from build123d import *

# Parameters (mm, degrees)
SKETCH6_R          = 4.25
CUT_EXTRUDE3_DEPTH = 20.176579466
CUT_EXTRUDE4_DEPTH = 6.35


with BuildPart() as part:
    # Sketch2 → Revolve1 (revolve)
    with BuildSketch(Plane(origin=(0, 0, 0), x_dir=(0, 0, -1), z_dir=(1, 0, 0)), mode=Mode.PRIVATE) as revolve1_sk:
        Polygon((0, 0), (-6.35, 0), (-10.16, -9.525), (-10.16, -12.7), (0, -12.7), align=None)
    revolve(revolve1_sk.sketch.rotate(Axis((0, -12.7, 0), (0, 1, 0)), 180), axis=Axis((0, -12.7, 0), (0, 1, 0)))

    # Sketch6 → Cut-Extrude3 (cut, through all)
    with BuildSketch(Plane(origin=(0, 0, 0), x_dir=(1, 0, 0), z_dir=(0, 1, 0))):
        with Locations(Location((0, 0, 0), (0, 0, 270))):
            Circle(SKETCH6_R)
    extrude(amount=-CUT_EXTRUDE3_DEPTH, mode=Mode.SUBTRACT)

    # Sketch7 → Cut-Extrude4 (cut)
    with BuildSketch(Plane.XZ.offset(12.7)):
        Polygon((0, 7.274613392), (-6.3, 3.637306696), (-6.3, -3.637306696), (0, -7.274613392), (6.3, -3.637306696), (6.3, 3.637306696), align=None)
    extrude(amount=-CUT_EXTRUDE4_DEPTH, mode=Mode.SUBTRACT)


solid = part.part
Verification items for the finished model (mm, model axes). A direction names the side the tool comes from. Give positions to 0.01 mm unless a question says otherwise; leave off trailing zeros. Loops run counter-clockwise (first coordinate to the right, second up) from the corner with the lowest first, then second, coordinate; pieces in that order, holes last.
1) Depth check by flat-ended pin: pin 1 Ø2 at (x, y) = (3, -3) entering from +Z; pin 2 Ø2 at (x, y) = (-2, -6.5) entering from +Z; pin 3 Ø6 at (y, z) = (-2.5, -2.5) entering from -X. Enter the tip coordinate at first touch or a pass-through.
2) Sectioned sample at A-A, the plane z = 0. Enter the section's corners in (x, y) (3 decimals).
3) Set-up check for faces 1 (the conical face through (-2.106, -1.654, -6.688)), 2 (the flat face through (3.194, -9.569, 5.43)): record each of +Z, -Z, +X, -X, +Y, -Y from which the full face is reachable in a straight line by a thin tool's end or side.
4) Sectioned sample at D-D, the plane y = -4.5. Enter the section's corners in (x, z), then the cut area to 3 significant figures.
5) Sectioned sample at C-C, the plane y = -8.25. Enter the section's corners in (x, z), then the cut area to 3 significant figures.
6) Draft check along X on faces 3 (the flat face through (-4, -6.35, -2)), 4 (the cylindrical face through (-10.074, -11.135, 1.323)), 5 (the flat face through (4, 0, -2)). Enter one of: pulls with the +X half, pulls with the -X half, needs draft (parallel to the pull), parting line crosses it, or undercut.
7) Thickness scan on line 1 along X through (y, z) = (-1.25, 0); line 2 along X through (y, z) = (-10.75, 7); line 3 along Y through (x, z) = (4.5, 4.25). Record the ranges inside material, lowest first.
8) Sectioned sample at B-B, the plane y = -10. Enter the section's corners in (x, z).
Answers:
1. pin 1: stops at z = 7.5
1. pin 2: stops at z = 9.18
1. pin 3: stops at x = -8.35
2. outline: (-10.16, -12.7) - (-6.3, -12.7) - (-6.3, -6.35) - (-4.25, -6.35) - (-4.25, 0) - (-6.35, 0) - (-10.16, -9.525) - close; (4.25, -6.35) - (6.3, -6.35) - (6.3, -12.7) - (10.16, -12.7) - (10.16, -9.525) - (6.35, 0) - (4.25, 0) - close
3. face 1: +Y
3. face 2: -Y
4. outline: circle Ø16.3 at (0, 0); hole circle Ø8.5 at (0, 0)
4. area: 152 mm2
5. outline: circle Ø19.3 at (0, 0); hole (-6.3, -3.64) - (0, -7.27) - (6.3, -3.64) - (6.3, 3.64) - (0, 7.27) - (-6.3, 3.64) - close
5. area: 155 mm2
6. face 3: undercut
6. face 4: parting line crosses it
6. face 5: needs draft
7. line 1: x = -6.85 to -4.25, 4.25 to 6.85
7. line 2: x = -7.36 to -0.48, 0.48 to 7.36
7. line 3: y = -6.35 to 0
8. outline: circle Ø20.32 at (0, 0); hole (-6.3, -3.64) - (0, -7.27) - (6.3, -3.64) - (6.3, 3.64) - (0, 7.27) - (-6.3, 3.64) - close
